```python
from build123d import *

# Parameters (mm, degrees)
SKETCH1_W                = 8
SKETCH1_H                = 1.2
SKETCH1_W_2              = 1
SKETCH1_H_2              = 4.1
REVOLVE1_ANGLE           = 180
SKETCH2_W                = 6.21
SKETCH2_H                = 1.5
CUT_EXTRUDE1_DEPTH       = 14.787313009
CUT_EXTRUDE2_DEPTH       = 14.787313009
SKETCH4_W                = 3.4
SKETCH4_H                = 2
BOSS_EXTRUDE1_DEPTH      = 1.2
SKETCH5_W                = 1.2
SKETCH5_H                = 2.9
BOSS_EXTRUDE2_DEPTH      = 1.5
CHAMFER1_SIZE            = 0.5
CHAMFER1_OF_MIRROR2_SIZE = 0.5
SKETCH6_W                = 2.8
SKETCH6_H                = 5
BOSS_EXTRUDE3_DEPTH      = 1.2
BOSS_EXTRUDE4_DEPTH      = 0.6


with BuildPart() as part:
    # Sketch1 → Revolve1 (revolve)
    with BuildSketch(Plane.XY):
        with Locations((4, 4.7)):
            Rectangle(SKETCH1_W, SKETCH1_H)
        with Locations((8.5, 4.7)):
            Rectangle(SKETCH1_W_2, SKETCH1_H)
        with Locations((8.5, 2.05)):
            Rectangle(SKETCH1_W_2, SKETCH1_H_2)
    revolve(axis=Axis((0, 0, 0), (0, 1, 0)), revolution_arc=REVOLVE1_ANGLE)

    # Sketch2 → Cut-Extrude1 (cut, through all)
    with BuildSketch(Plane.XY):
        with Locations((0, 3.35)):
            Rectangle(SKETCH2_W, SKETCH2_H)
    extrude(amount=-CUT_EXTRUDE1_DEPTH, mode=Mode.SUBTRACT)

    # Sketch3 → Cut-Extrude2 (cut, through all)
    with BuildSketch(Plane(origin=(0, 5.3, 0), x_dir=(1, 0, 0), z_dir=(0, 1, 0))):
        Polygon((-2.2, 5.8), (-3.6, 5.8), (-3.6, 0), (3.6, 0), (3.6, 5.8), (2.2, 5.8), (2.2, 0.8), (-2.2, 0.8), align=None)
    extrude(amount=-CUT_EXTRUDE2_DEPTH, mode=Mode.SUBTRACT)

    # Sketch4 → Boss-Extrude1 (add)
    with BuildSketch(Plane(origin=(0, 5.3, 0), x_dir=(1, 0, 0), z_dir=(0, 1, 0))):
        with Locations((5.3, -1)):
            Rectangle(SKETCH4_W, SKETCH4_H)
        with Locations((-5.3, -1)):
            Rectangle(SKETCH4_W, SKETCH4_H)
    extrude(amount=-BOSS_EXTRUDE1_DEPTH)

    # Sketch5 → Boss-Extrude2 (add)
    with BuildSketch(Plane(origin=(8, 0, 0), x_dir=(0, 0, -1), z_dir=(1, 0, 0))):
        with Locations((-0.6, 2.65)):
            Rectangle(SKETCH5_W, SKETCH5_H)
    boss_extrude2 = extrude(amount=BOSS_EXTRUDE2_DEPTH)

    # Chamfer1
    chamfer1_edges = [part.edges().sort_by_distance(p)[0] for p in [
        (9.5, 2.65, 1.2),
    ]]
    chamfer(chamfer1_edges, length=CHAMFER1_SIZE)

    # Mirror2: Boss-Extrude2 across plane
    add(boss_extrude2.mirror(Plane(origin=(0, 0, 0), x_dir=(0, 0, 1), z_dir=(1, 0, 0))))

    # Chamfer1 of Mirror2
    chamfer1_of_mirror2_edges = [part.edges().sort_by_distance(p)[0] for p in [
        (-9.5, 2.65, 1.2),
    ]]
    chamfer(chamfer1_of_mirror2_edges, length=CHAMFER1_OF_MIRROR2_SIZE)

    # Sketch6 → Boss-Extrude3 (add)
    with BuildSketch(Plane.XY.offset(-0.8)):
        with Locations((0, 7.8)):
            Rectangle(SKETCH6_W, SKETCH6_H)
    extrude(amount=-BOSS_EXTRUDE3_DEPTH)

    # Sketch7 → Boss-Extrude4 (add, symmetric)
    with BuildSketch(Plane(origin=(0, 0, 0), x_dir=(0, 0, -1), z_dir=(1, 0, 0))):
        Polygon((2, 10.3), (9, 5.3), (2, 5.3), align=None)
    extrude(amount=BOSS_EXTRUDE4_DEPTH, both=True)


solid = part.part
```
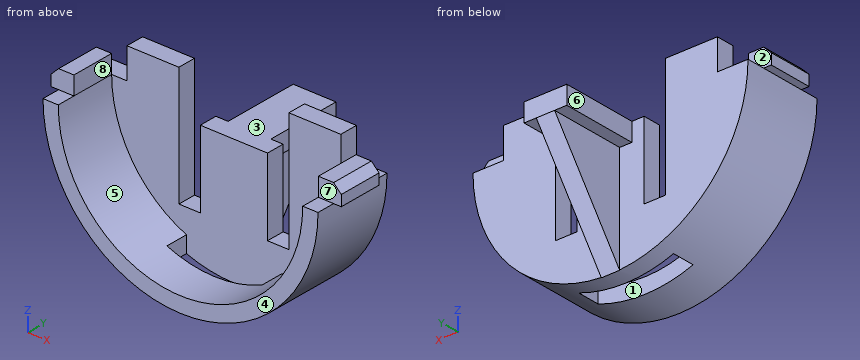
Work out the finished part from the listing and answer in its coordinate system (mm). Face numbers are marked on the shaded views. A direction names the side the tool comes from. Give positions to 0.01 mm unless a question says otherwise; leave off trailing zeros. Write each loop counter-clockwise with the first axis right and the second up, starting at its lowest first coordinate (ties: lowest second). Pieces come first, ordered by that corner, then holes. Notation, with made-up numbers: (40, -25.75) -> (70, -25.75) arc R25 cw to (70, 1.25) -> close; hole circle Ø11 at (89.25, 11). An arc over 180 degrees is marked (long way). Write item = value, one per line.
Q1. For a pull along Y with two mould halves and no side action, classify the marked faces 1, 2, 3 and 4 as pulls with the +Y half, pulls with the -Y half, needs draft (parallel to the pull), parting line crosses it, or undercut.
Computed values:
face_1 = undercut
face_2 = pulls with the +Y half
face_3 = needs draft
face_4 = pulls with the -Y half
Q2. Section B-B on z = -1.75 is taken. Determine the outline of the cut face in (x, y), and give its area (3 significant figures).
Computed values:
outline = (-8.83, 0) -> (-7.81, 0) -> (-7.81, 4.1) -> (-3.6, 4.1) -> (-3.6, 5.3) -> (-8.83, 5.3) -> close; (-2.2, 4.1) -> (2.2, 4.1) -> (2.2, 5.3) -> (1.4, 5.3) -> (1.4, 10.3) -> (-1.4, 10.3) -> (-1.4, 5.3) -> (-2.2, 5.3) -> close; (3.6, 4.1) -> (7.81, 4.1) -> (7.81, 0) -> (8.83, 0) -> (8.83, 5.3) -> (3.6, 5.3) -> close
area = 40.2 mm^2
Q3. Section D-D on y = 7.75 is taken. Determine the outline of the cut face in (x, z), and give its area (3 significant figures).
Computed values:
outline = (-1.4, -2) -> (-0.6, -2) -> (-0.6, -5.57) -> (0.6, -5.57) -> (0.6, -2) -> (1.4, -2) -> (1.4, -0.8) -> (-1.4, -0.8) -> close
area = 7.64 mm^2
Q4. Section A-A on y = 3.5 is taken. Determine the outline of the cut face in (x, z) (3 decimals).
Computed values:
outline = (-9.5, 0) -> (-9, 0) arc R9 ccw to (-3.105, -8.447) -> (-3.105, -7.373) arc R8 cw to (-8, 0) -> (-8, 1.2) -> (-9, 1.2) -> (-9.5, 0.7) -> close; (3.105, -8.447) arc R9 ccw to (9, 0) -> (9.5, 0) -> (9.5, 0.7) -> (9, 1.2) -> (8, 1.2) -> (8, 0) arc R8 cw to (3.105, -7.373) -> close
Q5. Consider line 1 along X through (y, z) = (7.5, -1.5); line 2 along X through (y, z) = (6.25, -3.25); line 3 along X through (y, z) = (4.5, -2). Determine where each line is inside the solid, lowest interval first.
Computed values:
line_1 = -1.4 to 1.4
line_2 = -0.6 to 0.6
line_3 = -8.77 to -3.6, -2.2 to 2.2, 3.6 to 8.77
Q6. Section C-C on z = -0.5 is taken. Determine the outline of the cut face in (x, y), and give its area (3 significant figures).
Computed values:
outline = (-8.99, 0) -> (-7.98, 0) -> (-7.98, 4.1) -> (-3.6, 4.1) -> (-3.6, 5.3) -> (-8.99, 5.3) -> close; (3.6, 4.1) -> (7.98, 4.1) -> (7.98, 0) -> (8.99, 0) -> (8.99, 5.3) -> (3.6, 5.3) -> close
area = 21.1 mm^2
Q7. Flat-ended cylindrical pins translate along their axes: pin 1 Ø3 at (y, z) = (2, -5) entering from -X; pin 2 Ø1 at (x, z) = (4.5, -6.5) entering from -Y; pin 3 Ø5 at (x, z) = (5, 0.5) entering from +Y; pin 4 Ø2 at (x, y) = (-1, 6.5) entering from +Z. Find the tip coordinate at first contact, or state that the pin passes through.
Computed values:
pin_1 = -8.29
pin_2 = 0
pin_3 = 5.3
pin_4 = -0.8
Q8. A tool of negligible diameter and unlimited length cuts with its end or side. For the marked faces 5, 6, 7 and 8, from which of +Z, -Z, +X, -X, +Y, -Y can it reach the whole face along a straight path? Write none if from no direction.
Computed values:
face_5 = +Z, -Y
face_6 = +Z, -Z, -X, +Y
face_7 = +Z, +X, -X, -Y
face_8 = +Z, +Y, -Y
